```python
from build123d import *

# Parameters (mm, degrees)
F0_W     = 50.8
F0_H     = 35.56
F1_DEPTH = 2.54
F3_DEPTH = 5.08


with BuildPart() as f1:
    # F0 (on Top) → F1 (new body)
    with BuildSketch(Plane.XY):
        Rectangle(F0_W, F0_H)
        with BuildLine():
            ThreePointArc((6.247574, 14.732), (0, -16.002), (-6.247574, 14.732))
            Line((-6.247574, 14.732), (6.247574, 14.732))
        make_face(mode=Mode.SUBTRACT)
    extrude(amount=F1_DEPTH)

    # F2 (on face) → F3 (join)
    with BuildSketch(Plane(origin=(0, 0, 0), x_dir=(1, 0, 0), z_dir=(0, 0, -1))):
        Polygon((-25.4, -17.78), (-22.86, -17.78), (-22.86, 15.24), (-16.51, 15.24), (-16.51, 17.78), (-25.4, 17.78), align=None)
        Polygon((22.86, -17.78), (25.4, -17.78), (25.4, 17.78), (16.51, 17.78), (16.51, 15.24), (22.86, 15.24), align=None)
    extrude(amount=F3_DEPTH)


solid = f1.part
```
Input: part model. Units: mm. Frame: model coordinates. A direction names the side the tool comes from. Coordinates: 2 decimals unless noted, no trailing zeros. Loops run counter-clockwise (first coordinate to the right, second up) from the corner with the lowest first, then second, coordinate; pieces in that order, holes last. Notation, with made-up numbers: M 55.5,12 L 93.5,12 A23 cw 93.5,41 Z; hole C 50.25,41.5 d10. An arc over 180 degrees is marked long. Use a Markdown table: item, result. Add a question column.
1) Section D-D, the plane x = -11. Return the cut outline in (y, z), plus the area to 3 significant figures.
2) Set-up query: faces 5 (the flat face through (-16.51, -16, -3)), 6 (the flat face through (-24, -4, -5.08)), 7 (the flat face through (22.86, 1, -3)). Return all of +Z, -Z, +X, -X, +Y, -Y with unobstructed straight access to the full face (end or side cutting, diameter ignored); none if empty.
3) Section A-A, the plane z = -3.25. Return the cut outline in (x, y).
4) Section B-B, the plane y = 0. Return the cut outline in (x, z), plus the area to 3 significant figures.
5) Draft query along Y for faces 1 (the flat face through (0.4, -17.78, 0.5)), 2 (the flat face through (0, 14.732, 1)), 3 (the flat face through (-20, -15.24, -3)), 4 (the flat face through (-22.86, 2, -3)). Return one class per face: +Y half, -Y half, draft (parallel to the pull), parting line (faces both ways), or undercut.
6) Section C-C, the plane x = 0. Return the cut outline in (y, z), plus the area to 3 significant figures.
7) Line query: L1, parallel to X at y = -5, z = -2; L2, parallel to Y at x = 0, z = 1.85; L3, parallel to X at y = 0, z = 1.65. Output: solid intervals per line, ascending. Write a range as from..to.
Answer below:
| question | item | result |
|---|---|---|
| 1 | outline | M -17.78,0 L -11.62,0 L -11.62,2.54 L -17.78,2.54 Z; M 11.62,0 L 17.78,0 L 17.78,2.54 L 11.62,2.54 Z |
| 1 | area | 31.3 mm2 |
| 2 | face 5 | -Z, +Y, -Y |
| 2 | face 6 | -Z, +X, -X, +Y, -Y |
| 2 | face 7 | -Z, +Y |
| 3 | outline | M -25.4,-17.78 L -16.51,-17.78 L -16.51,-15.24 L -22.86,-15.24 L -22.86,17.78 L -25.4,17.78 Z; M 16.51,-17.78 L 25.4,-17.78 L 25.4,17.78 L 22.86,17.78 L 22.86,-15.24 L 16.51,-15.24 Z |
| 4 | outline | M -25.4,-5.08 L -22.86,-5.08 L -22.86,0 L -16,0 L -16,2.54 L -25.4,2.54 Z; M 16,0 L 22.86,0 L 22.86,-5.08 L 25.4,-5.08 L 25.4,2.54 L 16,2.54 Z |
| 4 | area | 73.5 mm2 |
| 5 | face 1 | -Y half |
| 5 | face 2 | undercut |
| 5 | face 3 | +Y half |
| 5 | face 4 | draft |
| 6 | outline | M -17.78,0 L -16,0 L -16,2.54 L -17.78,2.54 Z; M 14.73,0 L 17.78,0 L 17.78,2.54 L 14.73,2.54 Z |
| 6 | area | 12.3 mm2 |
| 7 | L1 | -25.4..-22.86, 22.86..25.4 |
| 7 | L2 | -17.78..-16, 14.73..17.78 |
| 7 | L3 | -25.4..-16, 16..25.4 |
